For this review, take the finished solid that the model builds, in its own axes (mm). A direction names the side the tool comes from. Coordinates: 2 decimals unless noted, no trailing zeros. Loops run counter-clockwise (first coordinate to the right, second up) from the corner with the lowest first, then second, coordinate; pieces in that order, holes last. Notation, with made-up numbers: (15.25, 67) - (21.25, 67) arc R26 cw to (21.25, 102) - close; hole circle Ø10 at (62, -33.75). An arc over 180 degrees is marked (long way). Answer as a JSON object with one key per item and string values. Group by question number.
Item 1: We need section B-B (z = 0). Give the boundary of the cut face in (x, y).
Item 2: Mouldability with a two-part tool opening along Y and no side actions: class faces 1 (the cylindrical face through (0.126, 85.006, 0.55)), 2 (the flat face through (0, 51, -25)), 3 (the cylindrical face through (-32.53, -15.62, 3.47)) as released by +Y, released by -Y, zero draft, split by the parting line, or undercut.
Item 3: We need section C-C (x = -11.5). Give the boundary of the cut face in (y, z).
Item 4: We need section A-A (y = 0). Give the boundary of the cut face in (x, z), then the cut area to 3 significant figures.
Item 5: Clearance check with flat-ended pins moving along their axes: pin 1 (1 mm diameter, centred on x = 16, z = -13.5, fed in from +Y); pin 2 (10 mm diameter, centred on x = -7.5, z = 15, fed in from -Y); pin 3 (5 mm diameter, centred on y = 82.5, z = -12, fed in from -X). State where each tip first meets the part, or that it passes through.
Item 6: To check wall thickness, follow line 1 (X direction, y = 48.5, z = -11); line 2 (X direction, y = 26.5, z = -22); line 3 (Z direction, x = 32, y = -1). State the ranges of each line that lie inside material, in increasing order.
Item 7: Tool access review of faces 4 (the flat face through (-30, 33, 0)), 5 (the flat face through (20, 40, 0)), 6 (the flat face through (-30, 0, 0)), 7 (the flat face through (30, 0, 0)): name each direction out of +Z, -Z, +X, -X, +Y, -Y from which nothing blocks a thin tool from reaching the whole face with its end or side.
Item 8: We need section D-D (z = 10). Give the boundary of the cut face in (x, y), then the cut area to 3 significant figures.
from build123d import *

# Parameters (mm, degrees)
SKETCH1_R           = 28
SKETCH1_R_2         = 16
BOSS_EXTRUDE1_DEPTH = 35
BOSS_EXTRUDE2_DEPTH = 30
BOSS_EXTRUDE3_DEPTH = 9


with BuildPart() as part:
    # Sketch1 → Boss-Extrude1 (new, symmetric)
    with BuildSketch(Plane(origin=(0, 0, 0), x_dir=(0, 0, -1), z_dir=(1, 0, 0))):
        Circle(SKETCH1_R)
        Circle(SKETCH1_R_2, mode=Mode.SUBTRACT)
    extrude(amount=BOSS_EXTRUDE1_DEPTH, both=True)

    # Sketch2 → Boss-Extrude2 (add, symmetric)
    with BuildSketch(Plane(origin=(0, 0, 0), x_dir=(0, 0, -1), z_dir=(1, 0, 0))):
        with BuildLine():
            Line((-25, 40), (25, 40))
            Line((25, 40), (25, 12.609520213))
            ThreePointArc((25, 12.609520213), (0, -28), (-25, 12.609520213))
            Line((-25, 12.609520213), (-25, 40))
        make_face()
    extrude(amount=BOSS_EXTRUDE2_DEPTH, both=True)

    # Sketch3 → Boss-Extrude3 (add, symmetric)
    with BuildSketch(Plane(origin=(0, 0, 0), x_dir=(0, 0, -1), z_dir=(1, 0, 0))):
        with BuildLine():
            Line((-25, 40), (-25, 110))
            ThreePointArc((-25, 110), (0, 85), (25, 110))
            Line((25, 110), (25, 40))
            Line((25, 40), (25, 12.609520213))
            ThreePointArc((25, 12.609520213), (0, 28), (-25, 12.609520213))
            Line((-25, 12.609520213), (-25, 40))
        make_face()
    extrude(amount=BOSS_EXTRUDE3_DEPTH, both=True)


solid = part.part
Check sheet entries:
{
 "1": {"outline": "(-35, -28) - (35, -28) - (35, -16) - (30, -16) - (30, 16) - (35, 16) - (35, 28) - (30, 28) - (30, 40) - (9, 40) - (9, 85) - (-9, 85) - (-9, 40) - (-30, 40) - (-30, 28) - (-35, 28) - (-35, 16) - (-30, 16) - (-30, -16) - (-35, -16) - close"},
 "2": {"face 1": "released by +Y", "face 2": "zero draft", "face 3": "undercut"},
 "3": {"outline": "(12.61, -25) - (40, -25) - (40, 25) - (12.61, 25) arc R28 ccw (long way) to start"},
 "4": {"outline": "(-35, -28) - (35, -28) - (35, -16) - (30, -16) - (30, 16) - (35, 16) - (35, 28) - (-35, 28) - (-35, 16) - (-30, 16) - (-30, -16) - (-35, -16) - close", "area": "3,600 mm2"},
 "5": {"pin 1": "stops at y = 40", "pin 2": "stops at y = -26.15", "pin 3": "stops at x = -9"},
 "6": {"line 1": "x = -9 to 9", "line 2": "x = -30 to 30", "line 3": "z = -27.98 to -15.97, 15.97 to 27.98"},
 "7": {"face 4": "-X, +Y", "face 5": "+Z, -Z, +X, +Y", "face 6": "-X", "face 7": "+X"},
 "8": {"outline": "(-35, -26.15) - (35, -26.15) - (35, -12.49) - (30, -12.49) - (30, 12.49) - (35, 12.49) - (35, 26.15) - (30, 26.15) - (30, 40) - (9, 40) - (9, 87.09) - (-9, 87.09) - (-9, 40) - (-30, 40) - (-30, 26.15) - (-35, 26.15) - (-35, 12.49) - (-30, 12.49) - (-30, -12.49) - (-35, -12.49) - close", "area": "5,090 mm2"}
}
